Part print with two shaded views. Sizes in mm from the minimum x, y, z corner. A direction names the side the tool comes from. Give positions to 0.01 mm unless a question says otherwise; leave off trailing zeros. Write each loop counter-clockwise with the first axis right and the second up, starting at its lowest first coordinate (ties: lowest second). Pieces come first, ordered by that corner, then holes. Notation, with made-up numbers: (80, -33) -> (108, -33) arc R37 cw to (108, 5) -> close; hole circle Ø8 at (22.5, -12). An arc over 180 degrees is marked (long way). Answer in a Markdown table with one row per item. Add a question column.
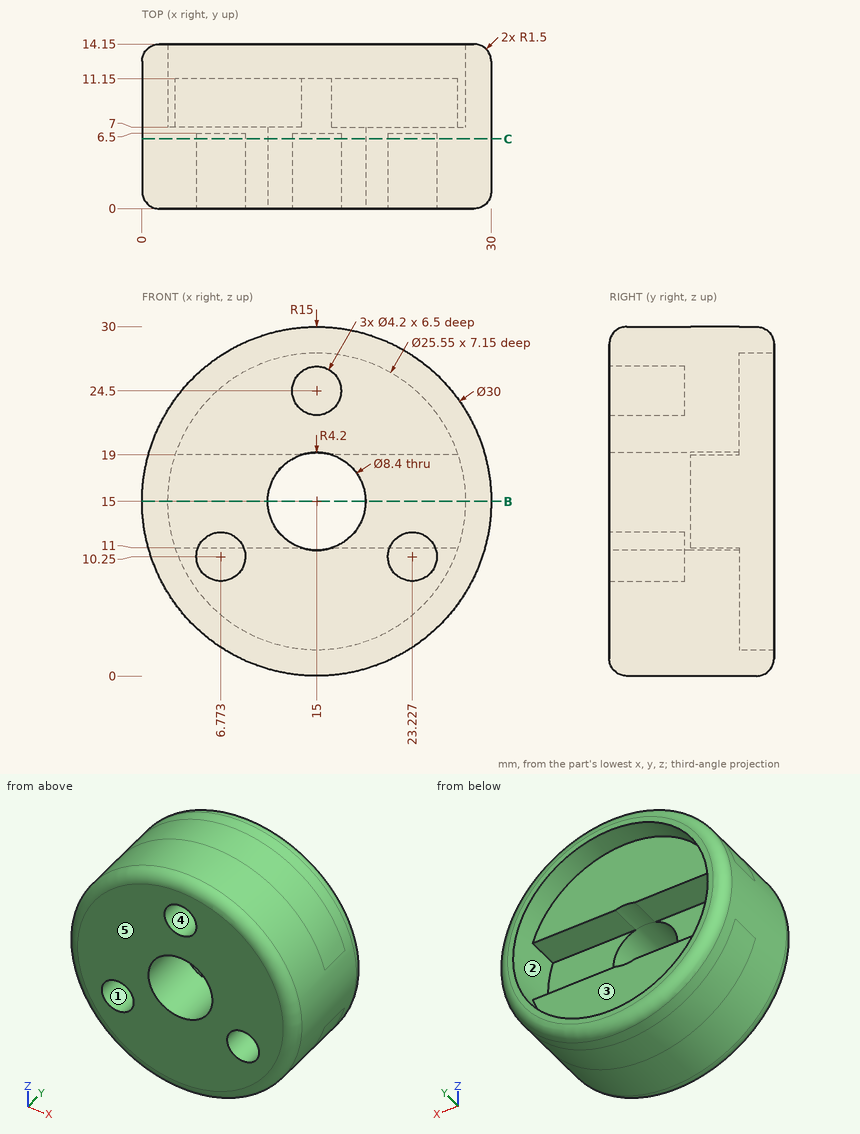
Item 1: Slice it at C-C, the plane y = 6. List the corners of the cut face in (x, z), then the cut area to 3 significant figures.
Item 2: Mould opens along X. For the marked faces 3, 4 and 5 say: released by +X, released by -X, zero draft, split by the parting line, or undercut.
Item 3: Which spindle directions (+Z, -Z, +X, -X, +Y, -Y) get a long thin tool onto all of the face, cutting with end or side? Do the marked faces 1 and 2. Say none if no direction does.
Item 4: Drop flat-ended pins along their axis: pin 1 Ø6 at (x, y) = (3.5, 7) entering from -Z; pin 2 Ø4 at (x, z) = (10.5, 15.5) entering from +Y; pin 3 Ø2 at (x, y) = (13, 7) entering from +Z. Give the stop position or say it passes through.
Item 5: Probe L1, parallel to X at y = 4, z = 15; L2, parallel to X at y = 5, z = 10.25; L3, parallel to X at y = 9, z = 15 (3 decimals). List the from-to ranges inside material, lowest first. Write a range as from..to.
Item 6: Slice it at B-B, the plane z = 15. List the corners of the cut face in (x, y) (3 decimals).
Answer key:
| question | item | result |
|---|---|---|
| 1 | outline | circle Ø30 at (15, 15); hole circle Ø4.2 at (6.77, 10.25); hole circle Ø8.4 at (15, 15); hole circle Ø4.2 at (15, 24.5); hole circle Ø4.2 at (23.23, 10.25) |
| 1 | area | 610 mm² |
| 2 | face 3 | undercut |
| 2 | face 4 | undercut |
| 2 | face 5 | zero draft |
| 3 | face 1 | -Y |
| 3 | face 2 | +Y |
| 4 | pin 1 | stops at z = 2.64 |
| 4 | pin 2 | stops at y = 7 |
| 4 | pin 3 | stops at z = 29.97 |
| 5 | L1 | x = 0..10.8, 19.2..30 |
| 5 | L2 | x = 0.77..4.67, 8.87..21.13, 25.33..29.23 |
| 5 | L3 | x = 0..2.225, 27.775..30 |
| 6 | outline | (0, 1.5) arc R1.5 ccw to (1.5, 0) -> (10.8, 0) -> (10.8, 7) -> (2.225, 7) -> (2.225, 14.15) -> (1.5, 14.15) arc R1.5 ccw to (0, 12.65) -> close; (19.2, 0) -> (28.5, 0) arc R1.5 ccw to (30, 1.5) -> (30, 12.65) arc R1.5 ccw to (28.5, 14.15) -> (27.775, 14.15) -> (27.775, 7) -> (19.2, 7) -> close |
